from build123d import *

# Parameters (mm, degrees)
F0_R     = 1.25
F1_DEPTH = 5
F2_R     = 2
F3_DEPTH = 4
F5_R     = 1


with BuildPart() as f1:
    # F0 (on Top) → F1 (new body)
    with BuildSketch(Plane.XY):
        with BuildLine():
            ThreePointArc((3.4551156036, 66.0154841021), (0, 68), (-3.4551156036, 66.0154841021))
            Line((-3.4551156036, 66.0154841021), (-38.4551156036, 6.0154841021))
            ThreePointArc((-38.4551156036, 6.0154841021), (-38.8613768538, 5.0439199169), (-39, 4))
            Line((-39, 4), (-39, 0))
            Line((-39, 0), (39, 0))
            Line((39, 0), (39, 4))
            ThreePointArc((39, 4), (38.8613768538, 5.0439199169), (38.4551156036, 6.0154841021))
            Line((38.4551156036, 6.0154841021), (3.4551156036, 66.0154841021))
        make_face()
        with BuildLine():
            Line((-29.4919272386, 5.5038710255), (-0.8637789009, 54.5806967473))
            ThreePointArc((-0.8637789009, 54.5806967473), (0, 55.0768257218), (0.8637789009, 54.5806967473))
            Line((0.8637789009, 54.5806967473), (29.4919272386, 5.5038710255))
            ThreePointArc((29.4919272386, 5.5038710255), (29.4952904903, 4.5019392735), (28.6281483377, 4))
            Line((28.6281483377, 4), (-28.6281483377, 4))
            ThreePointArc((-28.6281483377, 4), (-29.4952904903, 4.5019392735), (-29.4919272386, 5.5038710255))
        make_face(mode=Mode.SUBTRACT)
        with Locations((0, 64)):
            Circle(F0_R, mode=Mode.SUBTRACT)
    extrude(amount=F1_DEPTH)

    # F2 (on Front) → F3 (join)
    with BuildSketch(Plane.XZ):
        with BuildLine():
            Line((-39, 12), (-39, 0))
            Line((-39, 0), (-31, 0))
            Line((-31, 0), (-31, 12))
            ThreePointArc((-31, 12), (-31.8786796564, 14.1213203436), (-34, 15))
            Line((-34, 15), (-36, 15))
            ThreePointArc((-36, 15), (-38.1213203436, 14.1213203436), (-39, 12))
        make_face()
        with Locations((-35, 11)):
            Circle(F2_R, mode=Mode.SUBTRACT)
    extrude(amount=-F3_DEPTH)

    # F4: F1 across plane


with BuildPart() as f1_1:
    add(f1.part)
    add(f1.part.mirror(Plane.YZ))

    # F5
    f5_edges = [f1_1.edges().sort_by_distance(p)[0] for p in [
        (-35, 4, 5),
        (-31, 2, 5),
        (31, 2, 5),
        (35, 4, 5),
    ]]
    fillet(f5_edges, radius=F5_R)


solid = f1_1.part
Can you work these out from the model? Positions are in its coordinate system, mm. A direction names the side the tool comes from. Coordinates: 2 decimals unless noted, no trailing zeros. Write each loop counter-clockwise with the first axis right and the second up, starting at its lowest first coordinate (ties: lowest second). Pieces come first, ordered by that corner, then holes. Notation, with made-up numbers: (37, 65.25) - (43, 65.25) arc R31 cw to (43, 102.25) - close; hole circle Ø6 at (-24.5, 76.5). An arc over 180 degrees is marked (long way). Return JSON: item names as keys, results as strings. Group by question number.
Item 1: If we section it at C-C (x = 10.5): Write out the boundary of the cut face in (y, z), then the cut area to 3 significant figures.
Item 2: We'd pull the mould along Z, two halves only. Please class faces 1 (the face through (0, 4, 2)), 2 (the face through (33.092, 1.972, 11.601)), 3 (the face through (31.86, 1.97, 14.1)), 4 (the face through (-15, 32, 0)): pulls with the +Z half, pulls with the -Z half, needs draft (parallel to the pull), parting line crosses it, or undercut.
Item 3: If we section it at A-A (x = 0): Write out the boundary of the cut face in (y, z), then the cut area to 3 significant figures.
Item 4: I'm going to push flat-ended pins straight in: pin 1 Ø12 at (x, y) = (7.5, 36.5) entering from -Z; pin 2 Ø1.5 at (x, z) = (5, 4) entering from +Y; pin 3 Ø3 at (x, y) = (0, 64) entering from +Z. Where does each tip first touch, or does it pass through?
Item 5: Please list where this line runs through material, in increasing order: probe 1 along Z at (x, y) = (3.5, 64.5).
Item 6: If we section it at D-D (y = 7.5): Write out the boundary of the cut face in (x, z).
Item 7: Which directions (+Z, -Z, +X, -X, +Y, -Y) give clear straight access to the entire face, cutting with the end or side of a thin tool? Please do faces 5 (the face through (35, 2, 15)), 6 (the face through (-0.015, 55.077, 2.465)), 7 (the face through (35.1, 4, 8.6)).
Return value:
{
 "1": {"outline": "(0, 0) - (4, 0) - (4, 5) - (0, 5) - close; (38.06, 0) - (53.94, 0) - (53.94, 5) - (38.06, 5) - close", "area": "99.4 mm^2"},
 "2": {"face 1": "needs draft", "face 2": "undercut", "face 3": "pulls with the +Z half", "face 4": "pulls with the -Z half"},
 "3": {"outline": "(0, 0) - (4, 0) - (4, 5) - (0, 5) - close; (55.08, 0) - (62.75, 0) - (62.75, 5) - (55.08, 5) - close; (65.25, 0) - (68, 0) - (68, 5) - (65.25, 5) - close", "area": "72.1 mm^2"},
 "4": {"pin 1": "stops at z = 0", "pin 2": "stops at y = 64.65", "pin 3": "stops at z = 5"},
 "5": {"probe 1": "z = 0 to 5"},
 "6": {"outline": "(-37.59, 0) - (-28.33, 0) - (-28.33, 5) - (-37.59, 5) - close; (28.33, 0) - (37.59, 0) - (37.59, 5) - (28.33, 5) - close"},
 "7": {"face 5": "+Z, +X, -X, +Y, -Y", "face 6": "+Z, -Z", "face 7": "+Z, +X, -X, +Y"}
}
